Source: three-view drawing plus pictorial views. Frame: mm from the lowest corner of the part. A direction names the side the tool comes from. Coordinates: 2 decimals unless noted, no trailing zeros. Write each loop counter-clockwise with the first axis right and the second up, starting at its lowest first coordinate (ties: lowest second). Pieces come first, ordered by that corner, then holes. Notation, with made-up numbers: (-11.5, -25) -> (27.5, -25) arc R29 ccw to (27.5, 13) -> close; hole circle Ø3 at (-37, 37.25). An arc over 180 degrees is marked (long way). One line per item, written item: value. Start each with the question number.
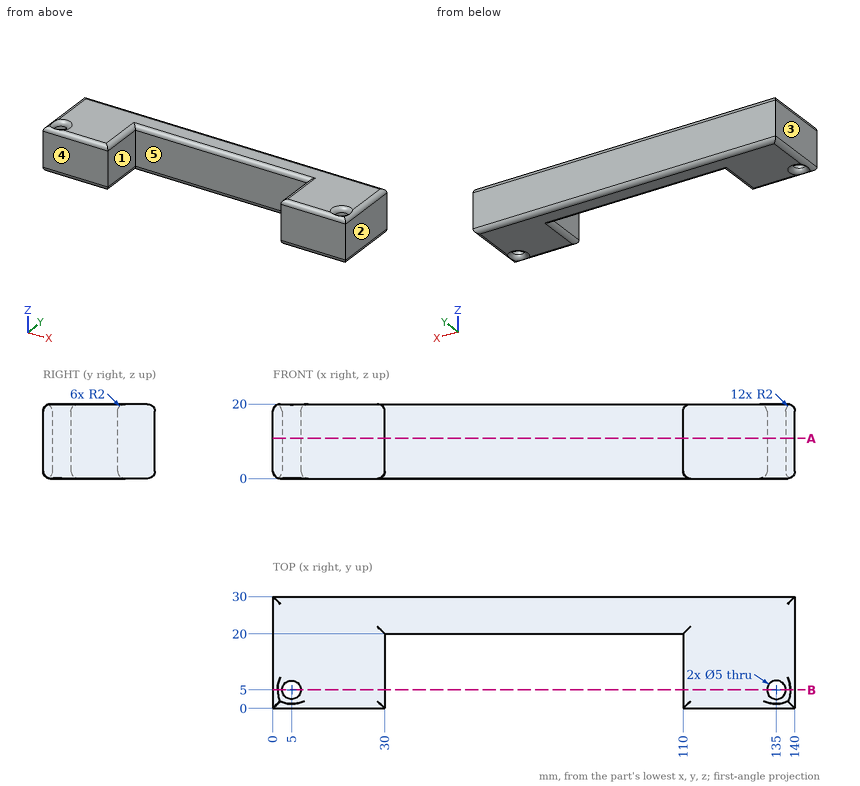
Q1. Cut plane B-B on y = 5. Count the separate pieces of the cut face and the enclosed holes in it, and give its area (3 significant figures).
Q2. Cut plane A-A on z = 10.75. Output: boundary loops of the cut face in (x, y), and give its area (3 significant figures).
Q3. Access query for the marked faces 1 and 2. Directions: +Z, -Z, +X, -X, +Y, -Y. A direction counts if a zero-diameter tool reaches every point of the face in a straight line with its end or side. Return the directions, or none.
Q4. First-contact query: P1, Ø4, axis at x = 5, y = 5, coming from the +Z side; P2, Ø6, axis at x = 135, y = 5, coming from the +Z side; P3, Ø10, axis at x = 99.5, z = 7.5, coming from the -Y side. Flat tips, straight axial feed; report the tip coordinate or a pass-through.
Q5. Line query: L1, parallel to X at y = 17, z = 7; L2, parallel to Y at x = 5, z = 6.5; L3, parallel to X at y = 3.5, z = 6. Output: solid intervals per line, ascending. Write a range as from..to.
Q6. Draft query along X for the marked faces 3, 4 and 5. Return one class per face: pulls with the +X half, pulls with the -X half, needs draft (parallel to the pull), parting line crosses it, or undercut.
Solution:
1. separate pieces: 4
1. enclosed holes: 0
1. area: 987 mm²
2. outline: (0, 0) -> (30, 0) -> (30, 20) -> (110, 20) -> (110, 0) -> (140, 0) -> (140, 30) -> (0, 30) -> close; hole circle Ø5 at (5, 5); hole circle Ø5 at (135, 5)
2. area: 2,560 mm²
3. face 1: +Z, -Z, -Y
3. face 2: +Z, -Z, +X, +Y, -Y
4. P1: through
4. P2: z = 19.32
4. P3: y = 20
5. L1: 0..30, 110..140
5. L2: 0..2.5, 7.5..30
5. L3: 0..3, 7..30, 110..133, 137..140
6. face 3: pulls with the -X half
6. face 4: needs draft
6. face 5: undercut
